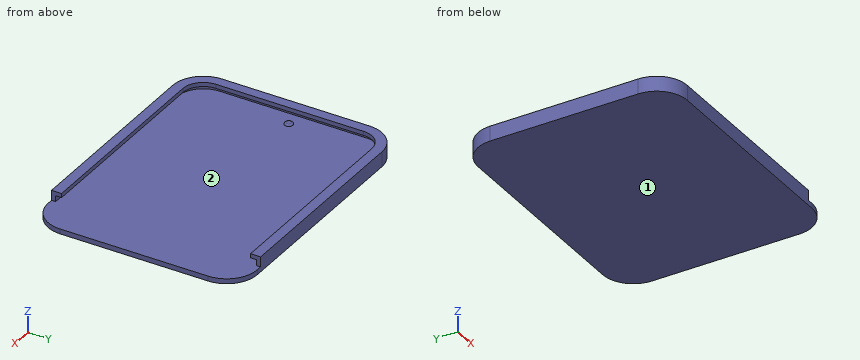
```python
from build123d import *

# Parameters (mm, degrees)
F1_DEPTH = 3.65
F3_DEPTH = 2.45
F5_DEPTH = 1
F6_W     = 11.5363439545
F6_H     = 60.74937433
F7_DEPTH = 25
F8_R     = 1
F9_DEPTH = 0.4
F10_R    = 0.39999


# Not quite as in the source:
# - a fillet or chamfer is up to 0.001 mm smaller than in the source, because OpenCascade refuses the exact size


with BuildPart() as f1:
    # F0 (on Top) → F1 (new body)
    with BuildSketch(Plane.XY):
        with BuildLine():
            ThreePointArc((-62.0253431911, -15.11933375), (-59.843288711, -20.3872792698), (-54.5753431911, -22.56933375))
            Line((-54.5753431911, -22.56933375), (-4.5753431911, -22.56933375))
            ThreePointArc((-4.5753431911, -22.56933375), (0.6926023287, -20.3872792698), (2.8746568089, -15.11933375))
            Line((2.8746568089, -15.11933375), (2.8746568089, 20.88066625))
            ThreePointArc((2.8746568089, 20.88066625), (0.6926023287, 26.1486117698), (-4.5753431911, 28.33066625))
            Line((-4.5753431911, 28.33066625), (-54.5753431911, 28.33066625))
            ThreePointArc((-54.5753431911, 28.33066625), (-59.843288711, 26.1486117698), (-62.0253431911, 20.88066625))
            Line((-62.0253431911, 20.88066625), (-62.0253431911, -15.11933375))
        make_face()
    extrude(amount=F1_DEPTH)

    # F2 (on face) → F3 (cut)
    with BuildSketch(Plane.XY.offset(3.65)):
        with BuildLine():
            Line((1.8746568089, -15.11933375), (1.8746568089, 20.88066625))
            ThreePointArc((1.8746568089, 20.88066625), (-0.0145044525, 25.4415049886), (-4.5753431911, 27.33066625))
            Line((-4.5753431911, 27.33066625), (-54.5753431911, 27.33066625))
            ThreePointArc((-54.5753431911, 27.33066625), (-59.1361819298, 25.4415049886), (-61.0253431911, 20.88066625))
            Line((-61.0253431911, 20.88066625), (-61.0253431911, -15.11933375))
            ThreePointArc((-61.0253431911, -15.11933375), (-59.1361819298, -19.6801724887), (-54.5753431911, -21.56933375))
            Line((-54.5753431911, -21.56933375), (-4.5753431911, -21.56933375))
            ThreePointArc((-4.5753431911, -21.56933375), (-0.0145044525, -19.6801724887), (1.8746568089, -15.11933375))
        make_face()
    extrude(amount=-F3_DEPTH, mode=Mode.SUBTRACT)

    # F4 (on face) → F5 (join)
    with BuildSketch(Plane.XY.offset(3.65)):
        with BuildLine():
            Line((1.8746568089, -15.11933375), (1.8746568089, 20.88066625))
            ThreePointArc((1.8746568089, 20.88066625), (-0.0145044525, 25.4415049886), (-4.5753431911, 27.33066625))
            Line((-4.5753431911, 27.33066625), (-54.5753431911, 27.33066625))
            ThreePointArc((-54.5753431911, 27.33066625), (-59.1361819298, 25.4415049886), (-61.0253431911, 20.88066625))
            Line((-61.0253431911, 20.88066625), (-61.0253431911, -15.11933375))
            ThreePointArc((-61.0253431911, -15.11933375), (-59.1361819298, -19.6801724887), (-54.5753431911, -21.56933375))
            Line((-54.5753431911, -21.56933375), (-4.5753431911, -21.56933375))
            ThreePointArc((-4.5753431911, -21.56933375), (-0.0145044525, -19.6801724887), (1.8746568089, -15.11933375))
        make_face()
        with BuildLine():
            ThreePointArc((-4.5753431911, 25.88066625), (-1.0398092852, 24.4162001559), (0.4246568089, 20.88066625))
            Line((0.4246568089, 20.88066625), (0.4246568089, -15.11933375))
            ThreePointArc((0.4246568089, -15.11933375), (-1.0398092852, -18.6548676559), (-4.5753431911, -20.11933375))
            Line((-4.5753431911, -20.11933375), (-54.5753431911, -20.11933375))
            ThreePointArc((-54.5753431911, -20.11933375), (-58.1108770971, -18.6548676559), (-59.5753431911, -15.11933375))
            Line((-59.5753431911, -15.11933375), (-59.5753431911, 20.88066625))
            ThreePointArc((-59.5753431911, 20.88066625), (-58.1108770971, 24.4162001559), (-54.5753431911, 25.88066625))
            Line((-54.5753431911, 25.88066625), (-4.5753431911, 25.88066625))
        make_face(mode=Mode.SUBTRACT)
    extrude(amount=-F5_DEPTH)

    # F6 (on face) → F7 (cut)
    with BuildSketch(Plane.XY.offset(1.2)):
        with Locations((-0.1405403018, 2.3494064808)):
            Rectangle(F6_W, F6_H)
    extrude(amount=F7_DEPTH, mode=Mode.SUBTRACT)

    # F8 (on face) → F9 (join)
    with BuildSketch(Plane.XY.offset(1.2)):
        with Locations((-57.3753431911, 3.9823222905)):
            Circle(F8_R)
    extrude(amount=F9_DEPTH)

    # F10 (radius 0.4 in the source; OpenCascade refuses exactly that, so slightly less here)
    f10_edges = [f1.edges().sort_by_distance(p)[0] for p in [
        (-58.375343, 3.982322, 1.6),
    ]]
    fillet(f10_edges, radius=F10_R)


solid = f1.part
```
Part model, mm, in its own coordinate system. Face numbers are marked on the shaded views. Give positions to 0.01 mm unless a question says otherwise; leave off trailing zeros. Loops run counter-clockwise (first coordinate to the right, second up) from the corner with the lowest first, then second, coordinate; pieces in that order, holes last. Notation, with made-up numbers: M 73.5,1 L 121.5,1 A6 cw 121.5,9 Z; hole C -8.75,-12.75 d2. An arc over 180 degrees is marked long. Return JSON: item names as keys, results as strings.
1) Pull direction Y, two halves, no side cores. Call the marked faces 1 and 2: released by +Y, released by -Y, zero draft, split by the parting line, or undercut.
Calculated:
{"face 1": "zero draft", "face 2": "undercut"}
2) Saw through at A-A, the plane y = -5. List the corners of the cut face in (x, z).
Calculated:
{"outline": "M -62.03,0 L 2.87,0 L 2.87,1.2 L -61.03,1.2 L -61.03,2.65 L -59.58,2.65 L -59.58,3.65 L -62.03,3.65 Z"}
3) Saw through at B-B, the plane x = -13. List the corners of the cut face in (y, z).
Calculated:
{"outline": "M -22.57,0 L 28.33,0 L 28.33,3.65 L 25.88,3.65 L 25.88,2.65 L 27.33,2.65 L 27.33,1.2 L -21.57,1.2 L -21.57,2.65 L -20.12,2.65 L -20.12,3.65 L -22.57,3.65 Z"}
4) Saw through at C-C, the plane y = -19. List the corners of the cut face in (x, z), then the cut area to 3 significant figures.
Calculated:
{"outline": "M -60.93,0 L 1.78,0 L 1.78,1.2 L -59.73,1.2 L -59.73,2.65 L -57.73,2.65 L -57.73,3.65 L -60.93,3.65 Z", "area": "80.2 mm2"}
5) Drill centre lines: line 1 (Y direction, x = -18.5, z = 1.45); line 2 (Y direction, x = -40.5, z = 3.4); line 3 (X direction, y = 13, z = 1.45). Where is each one in solid material? Low to high.
Calculated:
{"line 1": "y = -22.57 to -21.57, 27.33 to 28.33", "line 2": "y = -22.57 to -20.12, 25.88 to 28.33", "line 3": "x = -62.03 to -61.03"}
6) Flat gauge pins, fed straight in: pin 1 Ø24.5 at (x, y) = (-21, 1.5) entering from -Z; pin 2 Ø0.6 at (x, y) = (-57.5, 4) entering from +Z; pin 3 Ø10 at (x, y) = (-7, 9.5) entering from +Z; pin 4 Ø2 at (y, z) = (26.5, 2) entering from +X. Where does each tip first touch, or does it go through?
Calculated:
{"pin 1": "stops at z = 0", "pin 2": "stops at z = 1.6", "pin 3": "stops at z = 1.2", "pin 4": "stops at x = 0.93"}
